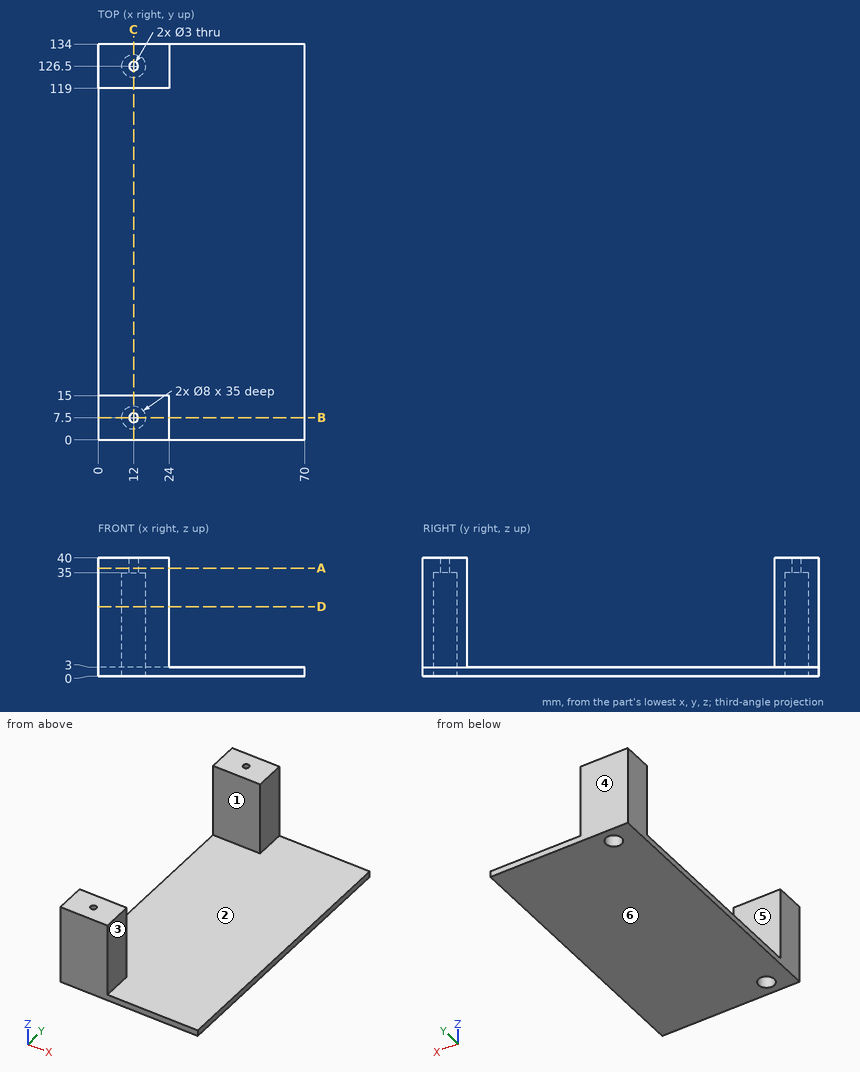
Geometry: see drawing. Coordinates: mm, zero at the bounding-box minimum. A direction names the side the tool comes from. Coordinates: 2 decimals unless noted, no trailing zeros. Loops run counter-clockwise (first coordinate to the right, second up) from the corner with the lowest first, then second, coordinate; pieces in that order, holes last. Notation, with made-up numbers: (-5.5, 44) -> (52.5, 44) arc R18 ccw to (52.5, 51) -> close; hole circle Ø3 at (1, -8). An arc over 180 degrees is marked (long way). Use a Markdown table: item, result.
1) Pull-direction query (Y, two-part tool) for the marked faces 4, 5 and 6; classes: released by +Y, released by -Y, zero draft, split by the parting line, or undercut.
Results found:
| item | result |
|---|---|
| face 4 | released by +Y |
| face 5 | undercut |
| face 6 | zero draft |
2) Access query for the marked faces 1, 2 and 3. Directions: +Z, -Z, +X, -X, +Y, -Y. A direction counts if a zero-diameter tool reaches every point of the face in a straight line with its end or side. Return the directions, or none.
Results found:
| item | result |
|---|---|
| face 1 | +Z, +X, -X |
| face 2 | +Z, +X |
| face 3 | +Z, +X, +Y, -Y |
3) Cut plane B-B (y = 7.5). Return the cut outline in (x, z), then the cut area to 3 significant figures.
Results found:
| item | result |
|---|---|
| outline | (0, 0) -> (8, 0) -> (8, 35) -> (10.5, 35) -> (10.5, 40) -> (0, 40) -> close; (13.5, 35) -> (16, 35) -> (16, 0) -> (70, 0) -> (70, 3) -> (24, 3) -> (24, 40) -> (13.5, 40) -> close |
| area | 803 mm2 |
4) Cut plane C-C (x = 12). Return the cut outline in (y, z).
Results found:
| item | result |
|---|---|
| outline | (0, 0) -> (3.5, 0) -> (3.5, 35) -> (6, 35) -> (6, 40) -> (0, 40) -> close; (9, 35) -> (11.5, 35) -> (11.5, 0) -> (122.5, 0) -> (122.5, 35) -> (125, 35) -> (125, 40) -> (119, 40) -> (119, 3) -> (15, 3) -> (15, 40) -> (9, 40) -> close; (128, 35) -> (130.5, 35) -> (130.5, 0) -> (134, 0) -> (134, 40) -> (128, 40) -> close |
5) Cut plane D-D (z = 23.5). Return the cut outline in (x, y).
Results found:
| item | result |
|---|---|
| outline | (0, 0) -> (24, 0) -> (24, 15) -> (0, 15) -> close; (0, 119) -> (24, 119) -> (24, 134) -> (0, 134) -> close; hole circle Ø8 at (12, 7.5); hole circle Ø8 at (12, 126.5) |
6) Material intervals for line 1 along Y through (x, z) = (12, 15); line 2 along Y through (x, z) = (12, 36.8); line 3 along Y through (x, z) = (21.5, 28), sorted ascending. Write a range as from..to.
Results found:
| item | result |
|---|---|
| line 1 | y = 0..3.5, 11.5..15, 119..122.5, 130.5..134 |
| line 2 | y = 0..6, 9..15, 119..125, 128..134 |
| line 3 | y = 0..15, 119..134 |
7) Cut plane A-A (z = 36.5). Return the cut outline in (x, y), then the cut area to 3 significant figures.
Results found:
| item | result |
|---|---|
| outline | (0, 0) -> (24, 0) -> (24, 15) -> (0, 15) -> close; (0, 119) -> (24, 119) -> (24, 134) -> (0, 134) -> close; hole circle Ø3 at (12, 7.5); hole circle Ø3 at (12, 126.5) |
| area | 706 mm2 |
8) Contact query for flat-ended pins moving along their axis: pin 1 (7 mm diameter, centred on x = 12, y = 126.5, fed in from -Z); pin 2 (16.5 mm diameter, centred on y = 10, z = 22, fed in from +X); pin 3 (4 mm diameter, centred on x = 58, y = 72, fed in from +Z). Output: stop coordinate, or through.
Results found:
| item | result |
|---|---|
| pin 1 | stops at z = 35 |
| pin 2 | stops at x = 24 |
| pin 3 | stops at z = 3 |
